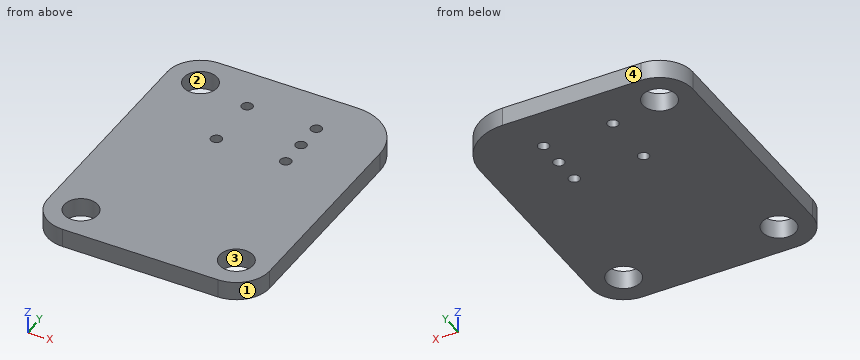
from build123d import *

# Parameters (mm, degrees)
BOARD_DEPTH        = 1.68
SKETCH2_R          = 1.5
SKETCH2_R_2        = 0.4953
PLATED_HOLES_DEPTH = 5.7


with BuildPart() as part:
    # Sketch1 → BOARD (new body)
    with BuildSketch(Plane.XY.offset(-4.7)):
        with BuildLine():
            Line((100, 42.5), (100, 60.5))
            ThreePointArc((100, 60.5), (98.681980515, 63.681980515), (95.5, 65))
            Line((95.5, 65), (83, 65))
            ThreePointArc((83, 65), (80.878679656, 64.121320344), (80, 62))
            Line((80, 62), (80, 42.5))
            ThreePointArc((80, 42.5), (80.878679656, 40.378679656), (83, 39.5))
            Line((83, 39.5), (97, 39.5))
            ThreePointArc((97, 39.5), (99.121320344, 40.378679656), (100, 42.5))
        make_face()
    extrude(amount=BOARD_DEPTH)

    # Sketch2 → PLATED HOLES (cut, through all)
    with BuildSketch(Plane.XY):
        with Locations((83, 42.5)):
            Circle(SKETCH2_R)
        with Locations((97, 42.5)):
            Circle(SKETCH2_R)
        with Locations((97, 35.5)):
            Circle(SKETCH2_R)
        with Locations((83, 62)):
            Circle(SKETCH2_R)
        with Locations((87.749999989, 55.999999989)):
            Circle(SKETCH2_R_2)
        with Locations((87.749999989, 60.999999996)):
            Circle(SKETCH2_R_2)
        with Locations((94.000000011, 58.499999992)):
            Circle(SKETCH2_R_2)
        with Locations((94.000000011, 55.999999989)):
            Circle(SKETCH2_R_2)
        with Locations((94.000000011, 60.999999996)):
            Circle(SKETCH2_R_2)
    extrude(amount=-PLATED_HOLES_DEPTH, mode=Mode.SUBTRACT)


solid = part.part
Could you check a few things on this model? Use its own coordinates, in mm. Face numbers are marked on the shaded views. Round coordinates to 2 decimals unless told otherwise and drop trailing zeros. Loops run counter-clockwise (first coordinate to the right, second up) from the corner with the lowest first, then second, coordinate; pieces in that order, holes last. Notation, with made-up numbers: (13, -4.75) - (67, -4.75) arc R29 cw to (67, 30.25) - close; hole circle Ø2 at (20.25, 89). An arc over 180 degrees is marked (long way). Write item = value, one per line.
1) Imagine slicing it at C-C (y = 61). Please give me the cut outline in (x, z), and give its area (3 significant figures).
Computed:
outline = (80, -4.7) - (81.88, -4.7) - (81.88, -3.02) - (80, -3.02) - close; (84.12, -4.7) - (87.25, -4.7) - (87.25, -3.02) - (84.12, -3.02) - close; (88.25, -4.7) - (93.5, -4.7) - (93.5, -3.02) - (88.25, -3.02) - close; (94.5, -4.7) - (99.97, -4.7) - (99.97, -3.02) - (94.5, -3.02) - close
area = 26.5 mm2
2) Imagine slicing it at B-B (z = -3.95). Give the number of separate pieces and of enclosed holes in the cut face, and give its area (3 significant figures).
Computed:
separate_pieces = 1
enclosed_holes = 8
area = 475 mm2
3) I need wall thicknesses on line 1 along Y through (x, z) = (83, -4.3); line 2 along Y through (x, z) = (94, -3.5); line 3 along X through (y, z) = (56, -3.85). Which ranges of each line are inside material? Lowest first, please. Write a range as from..to.
Computed:
line_1 = 39.5..41, 44..60.5, 63.5..65
line_2 = 39.5..55.5, 56.5..58, 59..60.5, 61.5..65
line_3 = 80..87.25, 88.25..93.5, 94.5..100
4) I'm going to push a flat-ended pin straight in: P1, Ø2.5, axis at x = 83, y = 62, coming from the +Z side. Where does the tip first touch, or does it pass through?
Computed:
P1 = through
5) Imagine slicing it at A-A (y = 56). Please give me the cut outline in (x, z), and give its area (3 significant figures).
Computed:
outline = (80, -4.7) - (87.25, -4.7) - (87.25, -3.02) - (80, -3.02) - close; (88.25, -4.7) - (93.5, -4.7) - (93.5, -3.02) - (88.25, -3.02) - close; (94.5, -4.7) - (100, -4.7) - (100, -3.02) - (94.5, -3.02) - close
area = 30.3 mm2
6) If we mould it in two halves opening along X, with no side actions, what happens to the marked faces 1, 2, 3 and 4? For each: pulls with the +X half, pulls with the -X half, needs draft (parallel to the pull), parting line crosses it, or undercut.
Computed:
face_1 = pulls with the +X half
face_2 = undercut
face_3 = undercut
face_4 = needs draft
